Autodesk Inventor part; units mm, degrees
ref_plane "YZ Plane" through (0, 0, 0) normal (1, 0, 0) x (0, 1, 0)
ref_plane "XZ Plane" through (0, 0, 0) normal (0, 1, 0) x (-1, 0, 0)
ref_plane "XY Plane" through (0, 0, 0) normal (0, 0, 1) x (1, 0, 0)
sketch "Skizze1" plane through (0, 0, 0) normal (0, 0, 1) x (1, 0, 0)
  line L0 (-4.424, 3.089) -> (90.576, 3.089)
  line L1 (90.576, 3.089) -> (90.576, -58.911)
  line L2 (90.576, -58.911) -> (-4.424, -58.911)
  line L3 (-4.424, -58.911) -> (-4.424, 3.089)
  line L4 (-1.424, 0.089) -> (87.576, 0.089)
  line L5 (87.576, 0.089) -> (87.576, -55.911)
  line L6 (87.576, -55.911) -> (-1.424, -55.911)
  line L7 (-1.424, -55.911) -> (-1.424, 0.089)
  point P0 (0, 0)
  dimension "d0" = 95
  dimension "d1" = 62
  dimension "d2" = 89
  dimension "d3" = 56
  dimension "d4" = 3
  dimension "d5" = 3
extrude "Extrusion1" add sketch "Skizze1" along normal blind 3 contours L0 L1 L2 L3 | L4 L5 L6 L7
sketch "Skizze2" plane through (0, 0, 3) normal (0, 0, 1) x (1, 0, 0)
  line L0 (90.576, 3.089) -> (-4.424, 3.089)
  line L1 (90.576, -58.911) -> (90.576, 3.089)
  line L2 (-4.424, 3.089) -> (90.576, 3.089)
  line L3 (90.576, 3.089) -> (90.576, -58.911)
  line L4 (90.576, -58.911) -> (-4.424, -58.911)
  line L5 (-4.424, -58.911) -> (-4.424, 3.089)
  line L6 (-4.424, 3.089) -> (90.576, 3.089)
  line L7 (90.576, 3.089) -> (90.576, -58.911)
  line L8 (90.576, -58.911) -> (-4.424, -58.911)
  line L9 (-4.424, -58.911) -> (-4.424, 3.089)
  line L10 (-1.424, 0.089) -> (87.576, 0.089)
  line L11 (87.576, 0.089) -> (87.576, -55.911)
  line L12 (87.576, -55.911) -> (-1.424, -55.911)
  line L13 (-1.424, -55.911) -> (-1.424, 0.089)
  point P0 (0, 0)
  point P1 (-4.124, -58.911)
  point P2 (4.776, -58.911)
  dimension "d8" = 89
  dimension "d9" = 56
  dimension "d10" = 3
  dimension "d11" = 3
extrude "Extrusion2" add sketch "Skizze2" along normal blind 56
fillet "Rundung1" radius 5 4 edges at (90.576, -58.911, 29.5) (90.576, 3.089, 29.5) (-4.424, -58.911, 29.5) (-4.424, 3.089, 29.5)
sketch "Skizze3" plane through (90.576, -53.911, 0) normal (1, 0, 0) x (0, 0, -1)
  line L0 (-38.1185, 15.5893) -> (-28.1185, 15.5893)
  line L1 (-28.1185, 15.5893) -> (-28.1185, 35.5893)
  line L2 (-28.1185, 35.5893) -> (-38.1185, 35.5893)
  line L3 (-38.1185, 35.5893) -> (-38.1185, 15.5893)
  point P0 (0, 53.911)
  dimension "d15" = 10
  dimension "d16" = 20
extrude "Extrusion3" cut sketch "Skizze3" against normal blind 100
fillet "Rundung2" radius 1 8 edges at (89.076, -38.3217, 28.1185) (89.076, -18.3217, 28.1185) (89.076, -18.3217, 38.1185) (89.076, -38.3217, 38.1185) (-2.924, -38.3217, 28.1185) (-2.924, -18.3217, 28.1185) (-2.924, -18.3217, 38.1185) (-2.924, -38.3217, 38.1185)
equation "\"d12\" = d9"
properties part number "bottom"
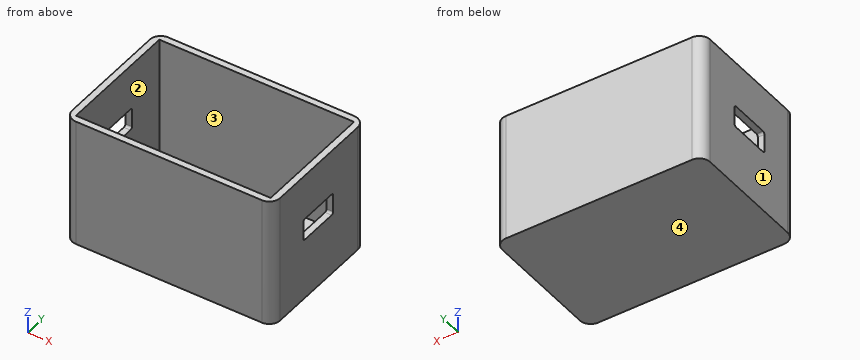
Geometry check sheet. Reference: the model listing, model coordinates, mm. Face numbers are marked on the shaded views. A direction names the side the tool comes from. Coordinates: 2 decimals unless noted, no trailing zeros. Order: outer loops, then holes, each group sorted by start corner. A loop starts at its lowest first (then second) coordinate and runs counter-clockwise, first axis right, second up. Notation, with made-up numbers: (89.5, 41) - (129.5, 41) arc R16 ccw to (129.5, 58) - close; hole circle Ø3 at (33.5, -17). An arc over 180 degrees is marked (long way). Answer in a Markdown table with one row per item. Add a question column.
1) Set-up check for the marked faces 1 and 2: record each of +Z, -Z, +X, -X, +Y, -Y from which the full face is reachable in a straight line by a thin tool's end or side.
2) Material ranges on line 1 along Y through (x, z) = (21, 44.5); line 2 along X through (y, z) = (-35, 53); line 3 along Z through (x, y) = (32.5, -11.5), recorded low to high. Write a range as [from, to].
3) Release check for a two-part mould opening along Z. For the marked faces 3 and 4 record: +Z half, -Z half, draft (parallel to the pull), parting line (faces both ways), or undercut.
4) Cross-section at C-C, the plane y = -33.5. Record the cut outline in (x, z), then the cut area to 3 significant figures.
5) Gauge pin test, flat ends, axial feed: P1, Ø2.5, axis at x = 89.5, y = -31.5, coming from the -Z side; P2, Ø1.5, axis at x = 89.5, z = 34, coming from the -Y side; P3, Ø3.5, axis at x = 89.5, z = 33, coming from the +Y side; P4, Ø2.5, axis at x = -2.5, z = 35, coming from the +Y side. Record the tip position at first contact, or that the pin passes through.
6) Cross-section at D-D, the plane x = 47. Record the cut outline in (y, z).
7) Cross-section at B-B, the plane z = 22. Record the cut outline in (x, y).
8) Cross-section at A-A, the plane z = 35. Record the cut outline in (x, y).
Check result:
| question | item | result |
|---|---|---|
| 1 | face 1 | +Z, -Z, -X, +Y, -Y |
| 1 | face 2 | +Z |
| 2 | line 1 | y = [-58.91, -55.91], [0.09, 3.09] |
| 2 | line 2 | x = [-4.42, -1.42], [87.58, 90.58] |
| 2 | line 3 | z = [0, 3] |
| 3 | face 3 | draft |
| 3 | face 4 | -Z half |
| 4 | outline | (-4.42, 0) - (90.58, 0) - (90.58, 28.12) - (87.58, 28.12) - (87.58, 3) - (-1.42, 3) - (-1.42, 28.12) - (-4.42, 28.12) - close; (-4.42, 38.12) - (-1.42, 38.12) - (-1.42, 59) - (-4.42, 59) - close; (87.58, 38.12) - (90.58, 38.12) - (90.58, 59) - (87.58, 59) - close |
| 4 | area | 561 mm² |
| 5 | P1 | stops at z = 0 |
| 5 | P2 | stops at y = -57.77 |
| 5 | P3 | stops at y = 2.59 |
| 5 | P4 | stops at y = 2.74 |
| 6 | outline | (-58.91, 0) - (3.09, 0) - (3.09, 59) - (0.09, 59) - (0.09, 3) - (-55.91, 3) - (-55.91, 59) - (-58.91, 59) - close |
| 7 | outline | (-4.42, -53.91) arc R5 ccw to (0.58, -58.91) - (85.58, -58.91) arc R5 ccw to (90.58, -53.91) - (90.58, -1.91) arc R5 ccw to (85.58, 3.09) - (0.58, 3.09) arc R5 ccw to (-4.42, -1.91) - close; hole (-1.42, -55.91) - (87.58, -55.91) - (87.58, 0.09) - (-1.42, 0.09) - close |
| 8 | outline | (-4.42, -53.91) arc R5 ccw to (0.58, -58.91) - (85.58, -58.91) arc R5 ccw to (90.58, -53.91) - (90.58, -38.32) - (87.58, -38.32) - (87.58, -55.91) - (-1.42, -55.91) - (-1.42, -38.32) - (-4.42, -38.32) - close; (-4.42, -18.32) - (-1.42, -18.32) - (-1.42, 0.09) - (87.58, 0.09) - (87.58, -18.32) - (90.58, -18.32) - (90.58, -1.91) arc R5 ccw to (85.58, 3.09) - (0.58, 3.09) arc R5 ccw to (-4.42, -1.91) - close |
